For this review, take the finished solid that the model builds, in its own axes (mm). Give positions to 0.01 mm unless a question says otherwise; leave off trailing zeros. Write each loop counter-clockwise with the first axis right and the second up, starting at its lowest first coordinate (ties: lowest second). Pieces come first, ordered by that corner, then holes. Notation, with made-up numbers: M 28.25,6 L 38.25,6 A7 ccw 38.25,11 Z; hole C 23.25,-18.5 d5. An arc over 180 degrees is marked long. Use one line per item in the form item = value. Start each with the question number.
Q1. Consider section D-D on z = 48. Write out the cut boundary in (x, y), and give its area (3 significant figures).
Q2. Consider section A-A on x = 31.5. Write out the cut boundary in (y, z).
Q3. For probe 1 along Y at (x, z) = (25, 304); probe 2 along X at (y, z) = (-26.5, 316.5) (3 decimals); probe 3 along X at (y, z) = (-34, 180.5) (3 decimals), list the stretches that pass through material, from the lowest coordinate up. Write a range as [from, to].
Q4. Consider section B-B on y = -6. Write out the cut boundary in (x, z), and give its area (3 significant figures).
Q5. Consider section C-C on z = 284. Write out the cut boundary in (x, y), and give its area (3 significant figures).
Q6. Clearance check with a flat-ended pin moving along its axis: pin 1 Ø4 at (y, z) = (-28.5, 71) entering from +X. State where the tip first meets the part, or that it passes through.
```python
from build123d import *

# Parameters (mm, degrees)
F1_DEPTH = 44.45
F3_DEPTH = 44.451


with BuildPart() as f1:
    # F0 (on Front) → F1 (new body)
    with BuildSketch(Plane.XZ):
        Polygon((0, 444.5), (0, 0), (25.4, 0), (44.45, 381), (44.45, 444.5), align=None)
    extrude(amount=F1_DEPTH)

    # F2 (on face) → F3 (cut, through all)
    with BuildSketch(Plane(origin=(0, 0, 0), x_dir=(0, -1, 0), z_dir=(-1, 0, 0))):
        Polygon((0, 381), (0, 0), (19.05, 0), align=None)
    extrude(amount=-F3_DEPTH, mode=Mode.SUBTRACT)


solid = f1.part
```
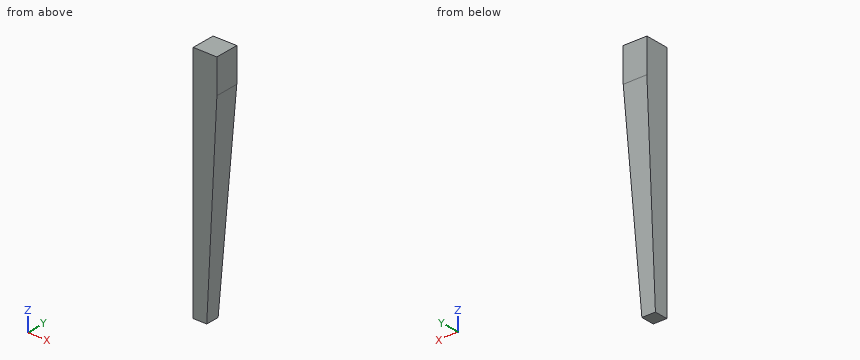
Working result:
q1.outline = M 0,-44.45 L 27.8,-44.45 L 27.8,-16.65 L 0,-16.65 Z
q1.area = 773 mm²
q2.outline = M -44.45,122 L -12.95,122 L 0,381 L 0,444.5 L -44.45,444.5 Z
q3.probe_1 = [-44.45, -3.85]
q3.probe_2 = [0, 41.225]
q3.probe_3 = [0, 34.425]
q4.outline = M 0,261 L 38.45,261 L 44.45,381 L 44.45,444.5 L 0,444.5 Z
q4.area = 7,800 mm²
q5.outline = M 0,-44.45 L 39.6,-44.45 L 39.6,-4.85 L 0,-4.85 Z
q5.area = 1,570 mm²
q6.pin_1 = 29.05
